Part model, mm, in its own coordinate system. Face numbers are marked on the shaded views. Give positions to 0.01 mm unless a question says otherwise; leave off trailing zeros. Write each loop counter-clockwise with the first axis right and the second up, starting at its lowest first coordinate (ties: lowest second). Pieces come first, ordered by that corner, then holes. Notation, with made-up numbers: M 13,39 L 30,39 A9 ccw 30,53 Z; hole C 1.5,19.25 d2. An arc over 180 degrees is marked long. Use a Markdown table: item, result.
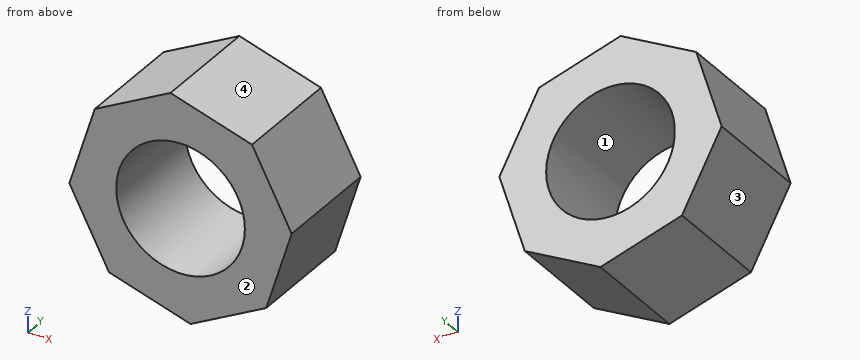
```python
from build123d import *

# Parameters (mm, degrees)
F0_R     = 14.725537
F1_DEPTH = 12.7


with BuildPart() as f1:
    # F0 (on Front) → F1 (new body, symmetric)
    with BuildSketch(Plane.XZ):
        Polygon((-19.607809, 16.352809), (-25.427997, -2.301632), (-16.352809, -19.607809), (2.301632, -25.427997), (19.607809, -16.352809), (25.427997, 2.301632), (16.352809, 19.607809), (-2.301632, 25.427997), align=None)
        Circle(F0_R, mode=Mode.SUBTRACT)
    extrude(amount=F1_DEPTH, both=True)


solid = f1.part
```
1. Cut at C-C, the plane x = 0. Give the cut face in (y, z).
Findings below:
| item | result |
|---|---|
| outline | M -12.7,-24.71 L 12.7,-24.71 L 12.7,-14.73 L -12.7,-14.73 Z; M -12.7,14.73 L 12.7,14.73 L 12.7,24.71 L -12.7,24.71 Z |
2. Drop flat-ended pins along their axis: P1, Ø5, axis at x = -15.5, y = 5, coming from the -Z side; P2, Ø8, axis at x = 11.5, y = -9.5, coming from the -Z side; P3, Ø23.5, axis at x = 0, z = 0, coming from the +Y side; P4, Ø6, axis at y = 3.5, z = 11, coming from the -X side. Give the stop position or say it passes through.
Findings below:
| item | result |
|---|---|
| P1 | z = -20.65 |
| P2 | z = -22.7 |
| P3 | through |
| P4 | x = -22.21 |
3. Cut at A-A, the plane y = -10.75. Give the cut face in (x, z).
Findings below:
| item | result |
|---|---|
| outline | M -25.43,-2.3 L -16.35,-19.61 L 2.3,-25.43 L 19.61,-16.35 L 25.43,2.3 L 16.35,19.61 L -2.3,25.43 L -19.61,16.35 Z; hole C 0,0 d29.45 |
4. Two-plate mould, pull along X, no slides. Class the marked faces 1, 2, 3 and 4: released by +X, released by -X, zero draft, split by the parting line, or undercut.
Findings below:
| item | result |
|---|---|
| face 1 | undercut |
| face 2 | zero draft |
| face 3 | released by -X |
| face 4 | released by +X |
5. Cut at B-B, the plane z = 0. Give the cut face in (x, y).
Findings below:
| item | result |
|---|---|
| outline | M -24.71,-12.7 L -14.73,-12.7 L -14.73,12.7 L -24.71,12.7 Z; M 14.73,-12.7 L 24.71,-12.7 L 24.71,12.7 L 14.73,12.7 Z |
6. Drill centre lines: L1, parallel to Z at x = 0, y = 5.5; L2, parallel to Z at x = -9, y = 8; L3, parallel to X at y = -6, z = -10. Where is each one in solid material? Low to high.
Findings below:
| item | result |
|---|---|
| L1 | -24.71 to -14.73, 14.73 to 24.71 |
| L2 | -21.9 to -11.66, 11.66 to 21.92 |
| L3 | -21.39 to -10.81, 10.81 to 21.59 |
